Autodesk Inventor part; units mm, degrees
ref_plane "YZ Plane" through (0, 0, 0) normal (1, 0, 0) x (0, 1, 0)
ref_plane "XZ Plane" through (0, 0, 0) normal (0, 1, 0) x (-1, 0, 0)
ref_plane "XY Plane" through (0, 0, 0) normal (0, 0, 1) x (1, 0, 0)
sketch "Sketch1" plane through (0, 0, 0) normal (0, 0, 1) x (1, 0, 0)
  circle A0 centre (0, 0) radius 4.7
  circle A1 centre (100, 0) radius 4.7
  circle A2 centre (0, 0) radius 9
  circle A3 centre (100, 0) radius 9
  line L0 (0, 9) -> (100, 9)
  line L1 (0, -9) -> (100, -9)
  dimension "d0" = 9.4
  dimension "d2" = 9.4
  dimension "d3" = 18
  dimension "d4" = 18
extrude "Extrusion1" add sketch "Sketch1" along normal blind 5
fillet "Fillet1" radius 0.5 8 edges at (50, -9, 5) (109, 0, 5) (50, 9, 5) (-9, 0, 5) (50, -9, 0) (109, 0, 0) (50, 9, 0) (-9, 0, 0)
fillet "Fillet2" radius 0.5 2 edges at (-4.7, 0, 5) (95.3, 0, 5)
properties part number "Arm Link Cross"
Design review of the part built by this model. Coordinates are the model's own, in mm. Give positions to 0.01 mm unless a question says otherwise; leave off trailing zeros. Loops run counter-clockwise (first coordinate to the right, second up) from the corner with the lowest first, then second, coordinate; pieces in that order, holes last. Notation, with made-up numbers: M -2.75,30 L 34.25,30 A20 cw 34.25,51 Z; hole C 78.5,9.5 d11. An arc over 180 degrees is marked long. Return JSON: item names as keys, results as strings. Group by question number.
Item 1: We need section A-A (y = 0). Give the boundary of the cut face in (x, z), and give its area (3 significant figures).
Item 2: We need section B-B (z = 3.2). Give the boundary of the cut face in (x, y), and give its area (3 significant figures).
Item 3: Insertion check: pin 1 Ø8.5 at (x, y) = (100, 0) entering from -Z. The pin has a flat end and moves straight along its axis. Give the tip position at first contact, or say it passes through.
Item 4: Mouldability with a two-part tool opening along X and no side actions: class faces 1 (the cylindrical face through (109, 0, 2)), 2 (the cylindrical face through (-1.02, 4.59, 2.22)), 3 (the cylindrical face through (-9, 0, 2)) as released by +X, released by -X, zero draft, split by the parting line, or undercut.
Item 5: For probe 1 along X at (y, z) = (-0.25, 3.45); probe 2 along Y at (x, z) = (100, 2.4); probe 3 along X at (y, z) = (-0.75, 2.1), list the stretches that pass through material, from the lowest coordinate up.
Output:
{
 "1": {"outline": "M -9,0.5 A0.5 ccw -8.5,0 L -4.7,0 L -4.7,4.5 A0.5 ccw -5.2,5 L -8.5,5 A0.5 ccw -9,4.5 Z; M 4.7,0 L 95.3,0 L 95.3,4.5 A0.5 ccw 94.8,5 L 5.2,5 A0.5 ccw 4.7,4.5 Z; M 104.7,0 L 108.5,0 A0.5 ccw 109,0.5 L 109,4.5 A0.5 ccw 108.5,5 L 105.2,5 A0.5 ccw 104.7,4.5 Z", "area": "496 mm^2"},
 "2": {"outline": "M 0,-9 L 100,-9 A9 ccw 100,9 L 0,9 A9 ccw Z; hole C 0,0 d9.4; hole C 100,0 d9.4", "area": "1,920 mm^2"},
 "3": {"pin 1": "passes through"},
 "4": {"face 1": "released by +X", "face 2": "undercut", "face 3": "released by -X"},
 "5": {"probe 1": "x = -9 to -4.69, 4.69 to 95.31, 104.69 to 109", "probe 2": "y = -9 to -4.7, 4.7 to 9", "probe 3": "x = -8.97 to -4.64, 4.64 to 95.36, 104.64 to 108.97"}
}
